```python
from build123d import *

# Parameters (mm, degrees)
SKETCH_1_W           = 70
SKETCH_1_H           = 18
EXTRUDE_1_DEPTH      = 60
CUT_EXTRUDE_1_DEPTH  = 94.936148527
SKETCH_3_W           = 15
SKETCH_3_H           = 5.3
CUT_EXTRUDE_2_DEPTH  = 1
SKETCH_4_W           = 15
SKETCH_4_H           = 5.3
CUT_EXTRUDE_3_DEPTH  = 1
SKETCH_5_W           = 3
SKETCH_5_H           = 11
CUT_EXTRUDE_4_DEPTH  = 1
SKETCH_6_W           = 3
SKETCH_6_H           = 11
CUT_EXTRUDE_5_DEPTH  = 1
CHAMFER_1_SIZE       = 1
EXTRUDE_9_DEPTH      = 6
SKETCH_7_W           = 29.5
SKETCH_7_H           = 9
CUT_EXTRUDE_7_DEPTH  = 4
SKETCH_9_W           = 37
SKETCH_9_H           = 7.5
EXTRUDE_3_DEPTH      = 12
SKETCH_10_W          = 70
SKETCH_10_H          = 18
EXTRUDE_4_DEPTH      = 8
CHAMFER_4_SIZE       = 4
SKETCH_11_W          = 8
SKETCH_11_H          = 11
CUT_EXTRUDE_8_DEPTH  = 3
SKETCH_12_W          = 0.6
SKETCH_12_H          = 33.5
CUT_EXTRUDE_9_DEPTH  = 13
SKETCH_13_W          = 0.6
SKETCH_13_H          = 52.5
EXTRUDE_5_DEPTH      = 6.7
SKETCH_14_W          = 0.6
SKETCH_14_H          = 10
EXTRUDE_6_DEPTH      = 1
SKETCH_15_W          = 7.7
SKETCH_15_H          = 49
EXTRUDE_7_DEPTH      = 0.6
SKETCH_18_W          = 7.7
SKETCH_18_H          = 10
EXTRUDE_8_DEPTH      = 0.6
CHAMFER_5_SIZE       = 1.8
SKETCH_22_W          = 3
SKETCH_22_H          = 6.5
CUT_EXTRUDE_10_DEPTH = 1
EXTRUDE_10_DEPTH     = 18
FILLET_1_R           = 3


with BuildPart() as part:
    # 草图1 → 凸台-拉伸1 (new body)
    with BuildSketch(Plane.XY):
        with Locations((35, 9)):
            Rectangle(SKETCH_1_W, SKETCH_1_H)
    extrude(amount=EXTRUDE_1_DEPTH)

    # 草图2 → 切除-拉伸1 (cut, through all)
    with BuildSketch(Plane.XY.offset(60)):
        Polygon((13.4, 0), (13.4, 5.3), (9.4, 5.3), (9.4, 12), (60.6, 12), (60.6, 5.3), (56.6, 5.3), (56.6, 0), align=None)
    extrude(amount=-CUT_EXTRUDE_1_DEPTH, mode=Mode.SUBTRACT)

    # 草图3 → 切除-拉伸2 (cut)
    with BuildSketch(Plane(origin=(13.4, 0, 0), x_dir=(0, 0, -1), z_dir=(1, 0, 0))):
        with Locations((-7.5, 2.65)):
            Rectangle(SKETCH_3_W, SKETCH_3_H)
    extrude(amount=-CUT_EXTRUDE_2_DEPTH, mode=Mode.SUBTRACT)

    # 草图4 → 切除-拉伸3 (cut)
    with BuildSketch(Plane.ZY.offset(-56.6)):
        with Locations((7.5, 2.65)):
            Rectangle(SKETCH_4_W, SKETCH_4_H)
    extrude(amount=-CUT_EXTRUDE_3_DEPTH, mode=Mode.SUBTRACT)

    # 草图5 → 切除-拉伸4 (cut)
    with BuildSketch(Plane(origin=(0, 5.3, 0), x_dir=(1, 0, 0), z_dir=(0, 1, 0))):
        with Locations((59.1, -5.5)):
            Rectangle(SKETCH_5_W, SKETCH_5_H)
    extrude(amount=-CUT_EXTRUDE_4_DEPTH, mode=Mode.SUBTRACT)

    # 草图6 → 切除-拉伸5 (cut)
    with BuildSketch(Plane(origin=(0, 5.3, 0), x_dir=(1, 0, 0), z_dir=(0, 1, 0))):
        with Locations((10.9, -5.5)):
            Rectangle(SKETCH_6_W, SKETCH_6_H)
    extrude(amount=-CUT_EXTRUDE_5_DEPTH, mode=Mode.SUBTRACT)

    # 倒角1
    chamfer_1_edges = [part.edges().sort_by_distance(p)[0] for p in [
        (59.1, 4.3, 11),
        (10.9, 4.3, 11),
        (12.4, 2.65, 15),
        (57.6, 2.65, 15),
    ]]
    chamfer(chamfer_1_edges, length=CHAMFER_1_SIZE - 0.0001)  # a hair under: the kernel refuses the full size

    # 草图21 → 凸台-拉伸9 (add)
    with BuildSketch(Plane(origin=(0, 18, 0), x_dir=(1, 0, 0), z_dir=(0, 1, 0))):
        Polygon((0, 0), (16.5, 8), (53.5, 8), (70, 0), align=None)
    extrude(amount=-EXTRUDE_9_DEPTH)

    # 草图7 → 切除-拉伸7 (cut)
    with BuildSketch(Plane.XZ.offset(-12)):
        with Locations((35, 0.5)):
            Rectangle(SKETCH_7_W, SKETCH_7_H)
    extrude(amount=-CUT_EXTRUDE_7_DEPTH, mode=Mode.SUBTRACT)

    # 草图9 → 凸台-拉伸3 (add)
    with BuildSketch(Plane.XZ.offset(-12)):
        with Locations((35, 56.25)):
            Rectangle(SKETCH_9_W, SKETCH_9_H)
    extrude(amount=EXTRUDE_3_DEPTH)

    # 草图10 → 凸台-拉伸4 (add)
    with BuildSketch(Plane.XY.offset(60)):
        with Locations((35, 9)):
            Rectangle(SKETCH_10_W, SKETCH_10_H)
    extrude(amount=EXTRUDE_4_DEPTH)

    # 倒角4
    chamfer_4_edges = [part.edges().sort_by_distance(p)[0] for p in [
        (35, 16, 5),
    ]]
    chamfer(chamfer_4_edges, length=CHAMFER_4_SIZE - 0.0001)  # a hair under: the kernel refuses the full size

    # 草图11 → 切除-拉伸8 (cut)
    with BuildSketch(Plane.XZ):
        with Locations((35, 58)):
            Rectangle(SKETCH_11_W, SKETCH_11_H)
    extrude(amount=-CUT_EXTRUDE_8_DEPTH, mode=Mode.SUBTRACT)

    # 草图12 → 切除-拉伸9 (cut)
    with BuildSketch(Plane.XZ):
        with Locations((22.5, 51.25)):
            Rectangle(SKETCH_12_W, SKETCH_12_H)
        with Locations((47.5, 51.25)):
            Rectangle(SKETCH_12_W, SKETCH_12_H)
    extrude(amount=-CUT_EXTRUDE_9_DEPTH, mode=Mode.SUBTRACT)

    # 草图13 → 凸台-拉伸5 (add)
    with BuildSketch(Plane.XZ.offset(-12)):
        with Locations((16.8, 26.25)):
            Rectangle(SKETCH_13_W, SKETCH_13_H)
        with Locations((53.2, 26.25)):
            Rectangle(SKETCH_13_W, SKETCH_13_H)
    extrude(amount=EXTRUDE_5_DEPTH)

    # 草图14 → 凸台-拉伸6 (add)
    with BuildSketch(Plane.XZ.offset(-5.3)):
        with Locations((16.8, 5)):
            Rectangle(SKETCH_14_W, SKETCH_14_H)
        with Locations((53.2, 5)):
            Rectangle(SKETCH_14_W, SKETCH_14_H)
    extrude(amount=EXTRUDE_6_DEPTH)

    # 草图15 → 凸台-拉伸7 (add)
    with BuildSketch(Plane.XZ.offset(-5.3)):
        with Locations((13.25, 35.5)):
            Rectangle(SKETCH_15_W, SKETCH_15_H)
        with Locations((56.75, 35.5)):
            Rectangle(SKETCH_15_W, SKETCH_15_H)
    extrude(amount=EXTRUDE_7_DEPTH)

    # 草图18 → 凸台-拉伸8 (add)
    with BuildSketch(Plane.XZ.offset(-4.3)):
        with Locations((13.25, 5)):
            Rectangle(SKETCH_18_W, SKETCH_18_H)
        with Locations((56.75, 5)):
            Rectangle(SKETCH_18_W, SKETCH_18_H)
    extrude(amount=EXTRUDE_8_DEPTH)

    # 倒角5
    chamfer_5_edges = [part.edges().sort_by_distance(p)[0] for p in [
        (35, 12, -8),
        (9.4, 12, 30),
        (60.6, 12, 30),
        (6.2, 0, 0),
        (63.8, 0, 0),
    ]]
    chamfer(chamfer_5_edges, length=CHAMFER_5_SIZE)

    # 草图22 → 切除-拉伸10 (cut)
    with BuildSketch(Plane.XZ):
        with Locations((24.3, 60.75)):
            Rectangle(SKETCH_22_W, SKETCH_22_H)
        with Locations((45.7, 60.75)):
            Rectangle(SKETCH_22_W, SKETCH_22_H)
    extrude(amount=-CUT_EXTRUDE_10_DEPTH, mode=Mode.SUBTRACT)

    # 草图23 → 凸台-拉伸10 (add)
    with BuildSketch(Plane(origin=(0, 18, 0), x_dir=(1, 0, 0), z_dir=(0, 1, 0))):
        Polygon((0, -68), (0, -86), (10, -86), (10, -83), (7, -83), (7, -79.7), (10, -79.7), (10, -76.7), (7, -76.7), (7, -68), align=None)
        Polygon((63, -68), (70, -68), (70, -86), (60, -86), (60, -83), (63, -83), (63, -79.7), (60, -79.7), (60, -76.7), (63, -76.7), align=None)
    extrude(amount=-EXTRUDE_10_DEPTH)

    # 圆角1
    fillet_1_edges = [part.edges().sort_by_distance(p)[0] for p in [
        (7, 9, 76.7),
        (7, 9, 68),
        (63, 9, 68),
        (63, 9, 76.7),
    ]]
    fillet(fillet_1_edges, radius=FILLET_1_R - 0.0001)  # a hair under: the kernel refuses the full size


solid = part.part
```
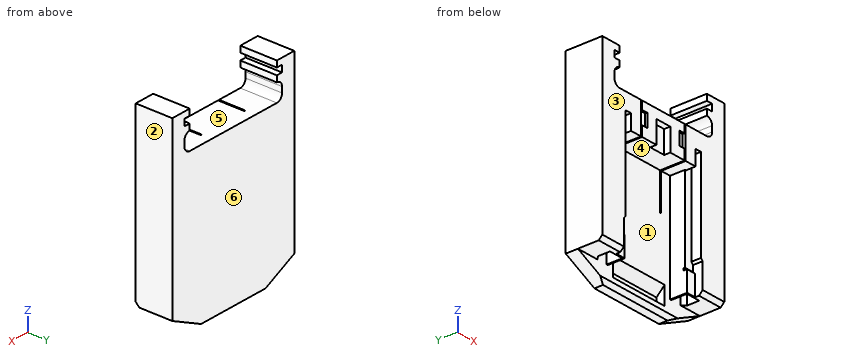
The model under review builds one solid part; all positions refer to its coordinate system, in mm. Face numbers are marked on the shaded views. A direction names the side the tool comes from. Give positions to 0.01 mm unless a question says otherwise; leave off trailing zeros. Write each loop counter-clockwise with the first axis right and the second up, starting at its lowest first coordinate (ties: lowest second). Pieces come first, ordered by that corner, then holes. Notation, with made-up numbers: M 40,44 L 55,44 A29 cw 55,73 Z; hole C -37,45.5 d8. An arc over 180 degrees is marked long. Write item = value, one per line. Start each with the question number.
Q1. We need section D-D (y = 8). Give the number of separate pieces and of enclosed holes in the cut face, plus the area to 3 significant figures.
Q2. For line 1 (X direction, y = 6, z = 31); line 2 (X direction, y = 10.5, z = 61); line 3 (Z direction, x = 9, y = 5.25), list the stretches that pass through material, from the lowest coordinate up.
Q3. Clearance check with flat-ended pins moving along their axes: pin 1 (0.8 mm diameter, centred on x = 46, y = 0.5, fed in from -Z); pin 2 (3.5 mm diameter, centred on x = 55.5, y = 2.5, fed in from -Z); pin 3 (0.7 mm diameter, centred on x = 47.5, y = 12.5, fed in from +Z). State where each tip first meets the part, or that it passes through.
Q4. Mouldability with a two-part tool opening along X and no side actions: class the marked faces 1, 2 and 3 as released by +X, released by -X, zero draft, split by the parting line, or undercut.
Q5. We need section A-A (z = 24). State the section outline as (x, y) points.
Q6. Machinability: for the marked faces 4, 5 and 6, which of the approach directions +Z, -Z, +X, -X, +Y, -Y give a long, thin tool a straight path to every point of the face, cutting with its end or side? Answer none if there is none.
Q7. We need section C-C (z = 75.5). State the section outline as (x, y) points, plus the area to 3 significant figures.
Result set:
q1.separate_pieces = 3
q1.enclosed_holes = 0
q1.area = 2,310 mm2
q2.line_1 = 0 to 9.4, 16.5 to 17.1, 52.9 to 53.5, 60.6 to 70
q2.line_2 = 0 to 22.2, 22.8 to 47.2, 47.8 to 70
q2.line_3 = 0 to 68.17, 76.53 to 79.7, 83 to 86
q3.pin_1 = 52.5
q3.pin_2 = 0
q3.pin_3 = 68
q4.face_1 = undercut
q4.face_2 = released by +X
q4.face_3 = zero draft
q5.outline = M 0,0 L 13.4,0 L 13.4,4.7 L 17.1,4.7 L 17.1,12 L 52.9,12 L 52.9,4.7 L 56.6,4.7 L 56.6,0 L 70,0 L 70,18 L 0,18 Z; hole M 9.4,5.3 L 16.5,5.3 L 16.5,12 L 11.2,12 L 9.4,10.2 Z; hole M 53.5,5.3 L 60.6,5.3 L 60.6,10.2 L 58.8,12 L 53.5,12 Z
q6.face_4 = -Z, -Y
q6.face_5 = +Z, +Y, -Y
q6.face_6 = +Z, -Z, +X, -X, +Y
q7.outline = M 0,0 L 7.6,0 L 7.6,18 L 0,18 Z; M 62.4,0 L 70,0 L 70,18 L 62.4,18 Z
q7.area = 274 mm2
